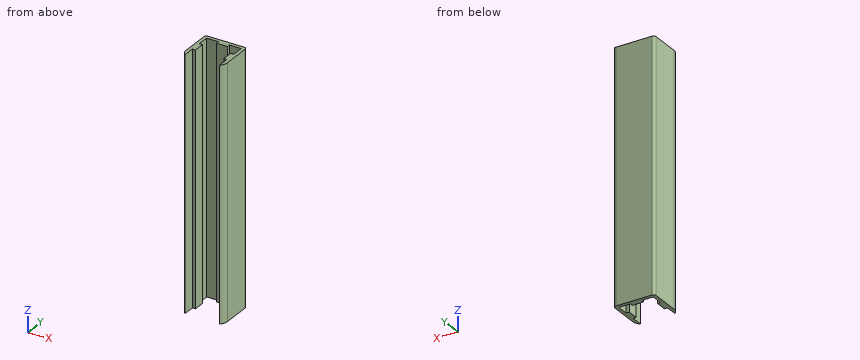
from build123d import *

# Parameters (mm, degrees)
F1_DEPTH    = 145
F2_T1_DEPTH = 165
F3_R        = 1.5


# Not quite as in the source:
# - a fillet or chamfer that OpenCascade refuses, or shapes differently, is made with other operations: its cross-section is extruded or revolved along the edge and cut away or added


with BuildPart() as f1:
    # F0 (on Top) → F1 (new body)
    with BuildSketch(Plane.XY):
        Polygon((8.4283615947, -32.4416384101), (10.4283615947, -32.4416384101), (10.4283615947, -25.6416384101), (12.2283615947, -25.6416384101), (12.2283615947, -19.2416384101), (10.4283615947, -19.2416384101), (10.4283615947, -12.4416384101), (17.2283615947, -12.4416384101), (17.2283615947, -14.2416384101), (23.6283615947, -14.2416384101), (23.6283615947, -12.4416384101), (30.4283615947, -12.4416384101), (30.4283615947, -19.2416384101), (28.6283615947, -19.2416384101), (28.6283615947, -25.6416384101), (30.4283615947, -25.6416384101), (30.4283615947, -32.4416384101), (32.4283615947, -32.4416384101), (32.4283615947, -10.4416384101), (8.4283615947, -10.4416384101), align=None)
    extrude(amount=F1_DEPTH)

    # F2: fillet of radius 5 on 2 edges, made by hand

    # F2_s2 → F2_t1 (cut)
    with BuildSketch(Plane.XY.offset(-10)):
        with BuildLine():
            ThreePointArc((8.4283615947, -28.4416384101), (8.9562256397, -30.6777063876), (10.4283615947, -32.4416384101))
            Line((10.4283615947, -32.4416384101), (8.4283615947, -32.4416384101))
            Line((8.4283615947, -32.4416384101), (8.4283615947, -28.4416384101))
        make_face()
        with BuildLine():
            ThreePointArc((30.4283615947, -32.4416384101), (31.9004975497, -30.6777063876), (32.4283615947, -28.4416384101))
            Line((32.4283615947, -28.4416384101), (32.4283615947, -32.4416384101))
            Line((32.4283615947, -32.4416384101), (30.4283615947, -32.4416384101))
        make_face()
    extrude(amount=F2_T1_DEPTH, mode=Mode.SUBTRACT)

    # F3
    f3_edges = [f1.edges().sort_by_distance(p)[0] for p in [
        (8.428362, -10.441638, 72.5),
        (32.428362, -10.441638, 72.5),
    ]]
    fillet(f3_edges, radius=F3_R)


solid = f1.part
Input: part model. Units: mm. Frame: model coordinates. Give positions to 0.01 mm unless a question says otherwise; leave off trailing zeros. Write each loop counter-clockwise with the first axis right and the second up, starting at its lowest first coordinate (ties: lowest second). Pieces come first, ordered by that corner, then holes. Notation, with made-up numbers: M -31.5,74.25 L -4.5,74.25 A11 cw -4.5,91.25 Z; hole C -38,-17 d9. An arc over 180 degrees is marked long. Use one line per item in the form item = value.
1. Cut plane C-C on x = 21.5. Return loops of the section in (y, z).
Outcome:
outline = M -14.24,0 L -10.44,0 L -10.44,145 L -14.24,145 Z
2. First-contact query: P1, Ø0.9, axis at x = 29.5, z = 65.5, coming from the -Y side; P2, Ø6, axis at x = 25.5, y = -20.5, coming from the -Z side; P3, Ø3.5, axis at x = 15, z = 49.5, coming from the -Y side; P4, Ø3, axis at x = 22, z = 39.5, coming from the -Y side. Flat tips, straight axial feed; report the tip coordinate or a pass-through.
Outcome:
P1 = -25.64
P2 = through
P3 = -12.44
P4 = -14.24
3. Cut plane B-B on z = 98. Return loops of the section in (x, y), and give its area (3 significant figures).
Outcome:
outline = M 8.43,-28.44 A5 ccw 10.43,-32.44 L 10.43,-25.64 L 12.23,-25.64 L 12.23,-19.24 L 10.43,-19.24 L 10.43,-12.44 L 17.23,-12.44 L 17.23,-14.24 L 23.63,-14.24 L 23.63,-12.44 L 30.43,-12.44 L 30.43,-19.24 L 28.63,-19.24 L 28.63,-25.64 L 30.43,-25.64 L 30.43,-32.44 A5 ccw 32.43,-28.44 L 32.43,-11.94 A1.5 ccw 30.93,-10.44 L 9.93,-10.44 A1.5 ccw 8.43,-11.94 Z
area = 157 mm²
4. Cut plane D-D on x = 15.25. Return loops of the section in (y, z), and give its area (3 significant figures).
Outcome:
outline = M -12.44,0 L -10.44,0 L -10.44,145 L -12.44,145 Z
area = 290 mm²
5. Ray query, L1, parallel to X at y = -14, z = 55.5; L2, parallel to X at y = -17, z = 42; L3, parallel to X at y = -23, z = 61.5. Return the intervals inside material, ascending.
Outcome:
L1 = 8.43 to 10.43, 17.23 to 23.63, 30.43 to 32.43
L2 = 8.43 to 10.43, 30.43 to 32.43
L3 = 8.43 to 12.23, 28.63 to 32.43
6. Cut plane A-A on y = -17. Return loops of the section in (x, z).
Outcome:
outline = M 8.43,0 L 10.43,0 L 10.43,145 L 8.43,145 Z; M 30.43,0 L 32.43,0 L 32.43,145 L 30.43,145 Z
